from build123d import *

# Parameters (mm, degrees)
FILLET1_R = 0.5


with BuildPart() as part:
    # Sketch1 → Revolve1 (revolve)
    with BuildSketch(Plane.XY):
        with BuildLine():
            Line((-1.5, 1), (1.5, 1))
            Line((1.5, 1), (1.5, 4.5))
            Line((1.5, 4.5), (2.25, 5.75))
            Line((2.25, 5.75), (2.25, 8.25))
            Line((2.25, 8.25), (1.5, 8.25))
            Line((1.5, 8.25), (1.5, 7.25))
            ThreePointArc((1.5, 7.25), (1.426776695, 7.073223305), (1.25, 7))
            Line((1.25, 7), (-1.25, 7))
            ThreePointArc((-1.25, 7), (-1.426776695, 7.073223305), (-1.5, 7.25))
            Line((-1.5, 7.25), (-1.5, 8.25))
            Line((-1.5, 8.25), (-2.25, 8.25))
            Line((-2.25, 8.25), (-2.25, 5.75))
            Line((-2.25, 5.75), (-1.5, 4.5))
            Line((-1.5, 4.5), (-1.5, 1))
        make_face()
    revolve(axis=Axis((0, 0, 0), (1, 0, 0)))

    # Fillet1
    fillet1_edges = [part.edges().sort_by_distance(p)[0] for p in [
        (-1.5, -8.25, 0),
        (1.5, -8.25, 0),
    ]]
    fillet(fillet1_edges, radius=FILLET1_R)


solid = part.part
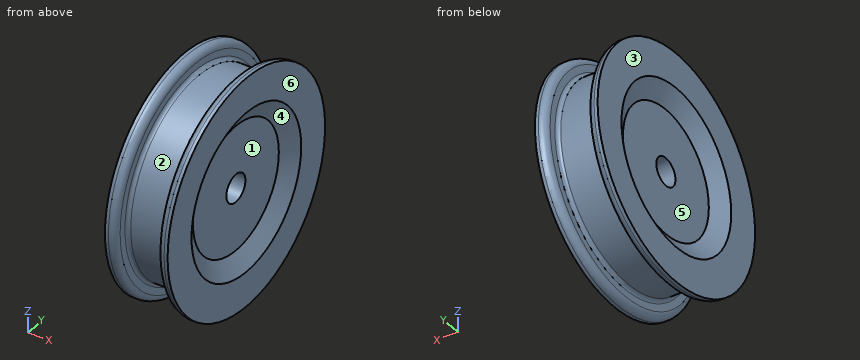
Can you work these out from the model? Positions are in its coordinate system, mm. Face numbers are marked on the shaded views. A direction names the side the tool comes from. Coordinates: 2 decimals unless noted, no trailing zeros. Write each loop counter-clockwise with the first axis right and the second up, starting at its lowest first coordinate (ties: lowest second). Pieces come first, ordered by that corner, then holes. Notation, with made-up numbers: M -24.5,74.5 L 26.5,74.5 A23 cw 26.5,98.5 Z; hole C 35,-38 d4. An arc over 180 degrees is marked long. Use one line per item in the form item = value.
Q1. I need wall thicknesses on line 1 along Z through (x, y) = (0.45, 0); line 2 along X through (y, z) = (-6.25, 3.75); line 3 along X through (y, z) = (0, 3.25). Which ranges of each line are inside material? Lowest first, please. Write a range as from..to.
Model answer:
line_1 = -7..-1, 1..7
line_2 = -2.25..-1.5, 1.5..2.25
line_3 = -1.5..1.5
Q2. For the marked faces 5 and 6, which set-ups out of +Z, -Z, +X, -X, +Y, -Y let a thin tool reach every point of the face, with its end or its side?
Model answer:
face_5 = -X
face_6 = +Z, -Z, +X, +Y, -Y
Q3. We'd pull the mould along Y, two halves only. Please class the marked faces 1, 2, 3 and 4: +Y half, -Y half, draft (parallel to the pull), parting line (faces both ways), or undercut.
Model answer:
face_1 = undercut
face_2 = parting line
face_3 = draft
face_4 = undercut
Q4. For P1, Ø3, axis at y = 0, z = 0, coming from the -X side; P2, Ø5, axis at y = 0.5, z = -1, coming from the +X side; P3, Ø8, axis at y = -0.5, z = -1.5, coming from the -X side, each with a flat end and sliding along its axis, tell me the tip position at first contact or that it passes through.
Model answer:
P1 = -1.5
P2 = 1.5
P3 = -2.15
Q5. If we section it at C-C (x = -0.7): Write out the boundary of the cut face in (y, z).
Model answer:
outline = C 0,0 d14; hole C 0,0 d2
